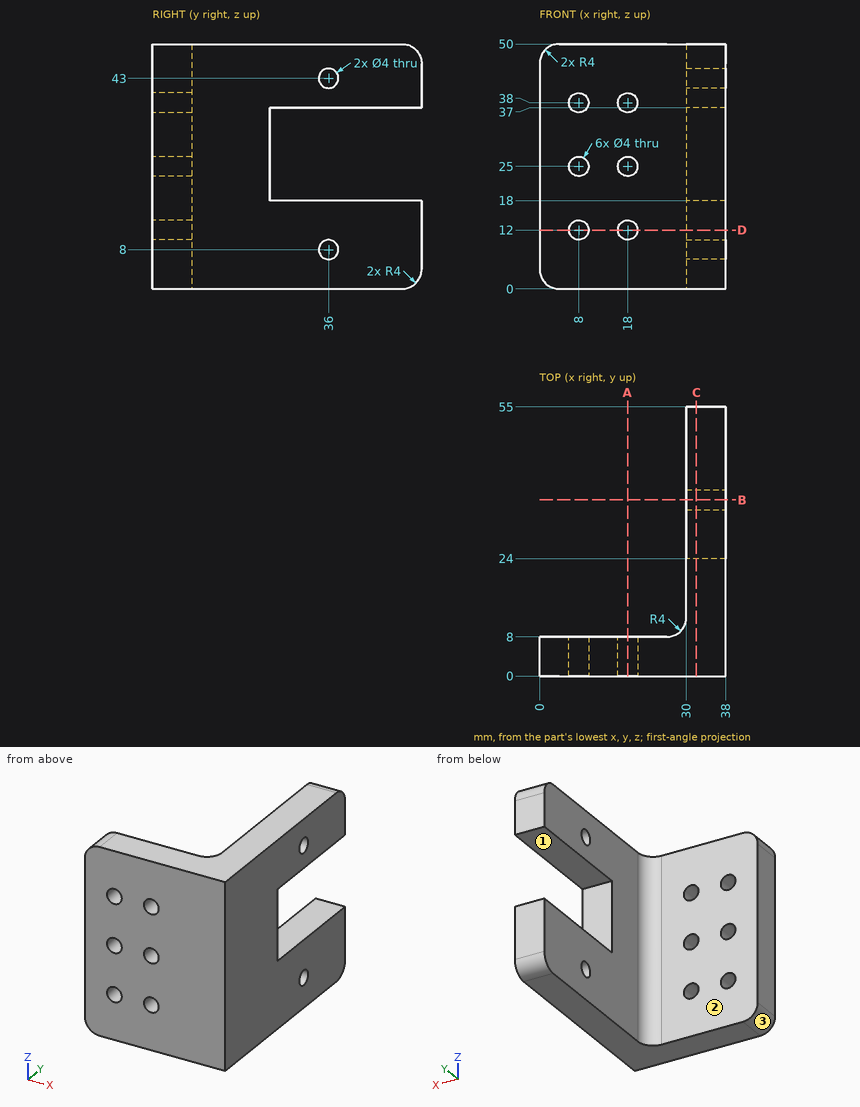
Geometry: see drawing. Coordinates: mm, zero at the bounding-box minimum. A direction names the side the tool comes from. Round coordinates to 2 decimals unless told otherwise and drop trailing zeros. Loops run counter-clockwise (first coordinate to the right, second up) from the corner with the lowest first, then second, coordinate; pieces in that order, holes last. Notation, with made-up numbers: M -1.5,-7.75 L 46.5,-7.75 A17 cw 46.5,4.25 Z; hole C -4,55 d7. An arc over 180 degrees is marked long. Use a Markdown table: item, result. Add a question column.
1. Ray query, line 1 along Z through (x, y) = (8, 6.5); line 2 along X through (y, z) = (46, 45); line 3 along Y through (x, z) = (6.5, 40.5). Return the intervals inside material, ascending. Write a range as [from, to].
2. Cut plane C-C, the plane x = 32. Output: boundary loops of the cut face in (y, z).
3. Contact query for flat-ended pins moving along their axis: pin 1 (12 mm diameter, centred on y = 23, z = 15, fed in from -X); pin 2 (5 mm diameter, centred on x = 8, z = 38, fed in from +Y); pin 3 (2.5 mm diameter, centred on x = 35.5, z = 25, fed in from +Y). Output: stop coordinate, or through.
4. Cut plane B-B, the plane y = 36. Output: boundary loops of the cut face in (x, z), and give its area (3 significant figures).
5. Cut plane D-D, the plane z = 12. Output: boundary loops of the cut face in (x, y), and give its area (3 significant figures).
6. Set-up query: the marked faces 1, 2 and 3. Return all of +Z, -Z, +X, -X, +Y, -Y with unobstructed straight access to the full face (end or side cutting, diameter ignored); none if empty.
7. Cut plane A-A, the plane x = 18. Output: boundary loops of the cut face in (y, z).
Solution:
| question | item | result |
|---|---|---|
| 1 | line 1 | z = [0, 10], [14, 23], [27, 36], [40, 50] |
| 1 | line 2 | x = [30, 38] |
| 1 | line 3 | y = [0, 8] |
| 2 | outline | M 0,0 L 51,0 A4 ccw 55,4 L 55,18 L 24,18 L 24,37 L 55,37 L 55,46 A4 ccw 51,50 L 0,50 Z; hole C 36,8 d4; hole C 36,43 d4 |
| 3 | pin 1 | stops at x = 30 |
| 3 | pin 2 | stops at y = 8 |
| 3 | pin 3 | stops at y = 24 |
| 4 | outline | M 30,0 L 38,0 L 38,6 L 30,6 Z; M 30,10 L 38,10 L 38,18 L 30,18 Z; M 30,37 L 38,37 L 38,41 L 30,41 Z; M 30,45 L 38,45 L 38,50 L 30,50 Z |
| 4 | area | 184 mm2 |
| 5 | outline | M 0,0 L 6,0 L 6,8 L 0,8 Z; M 10,0 L 16,0 L 16,8 L 10,8 Z; M 20,0 L 38,0 L 38,55 L 30,55 L 30,12 A4 cw 26,8 L 20,8 Z |
| 5 | area | 619 mm2 |
| 6 | face 1 | +X, -X, +Y |
| 6 | face 2 | +Z, -Z, -X, +Y |
| 6 | face 3 | -Z, -X, +Y, -Y |
| 7 | outline | M 0,0 L 8,0 L 8,10 L 0,10 Z; M 0,14 L 8,14 L 8,23 L 0,23 Z; M 0,27 L 8,27 L 8,36 L 0,36 Z; M 0,40 L 8,40 L 8,50 L 0,50 Z |
